Geometry: final body of the model. Coordinates: model frame, mm. Face numbers are marked on the shaded views. A direction names the side the tool comes from. Give positions to 0.01 mm unless a question says otherwise; leave off trailing zeros. Loops run counter-clockwise (first coordinate to the right, second up) from the corner with the lowest first, then second, coordinate; pieces in that order, holes last. Notation, with made-up numbers: (66.25, 24) - (79.25, 24) arc R24 cw to (79.25, 63) - close; hole circle Ø7 at (-9, 83). An arc over 180 degrees is marked (long way). Answer in a Markdown table with one row per item.
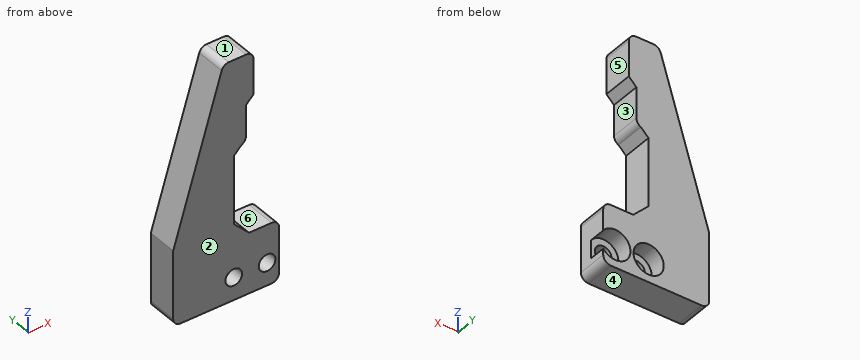
from build123d import *

# Parameters (mm, degrees)
BOSS_EXTRUDE1_DEPTH                                 = 10
CHAMFER1_SIZE                                       = 5
CHAMFER2_SIZE                                       = 2.5
FILLET1_R                                           = 2.5
CBORE_FOR_M5_HEX_SOCKET_HEAD_CAP_SCREW2_D           = 5.5
CBORE_FOR_M5_HEX_SOCKET_HEAD_CAP_SCREW2_DEPTH       = 10
CBORE_FOR_M5_HEX_SOCKET_HEAD_CAP_SCREW2_CBORE_D     = 10
CBORE_FOR_M5_HEX_SOCKET_HEAD_CAP_SCREW2_CBORE_DEPTH = 5.4
CBORE_FOR_M5_HEX_SOCKET_HEAD_CAP_SCREW2_TIP         = 1.652366702


# Some blends are built 0.0001 mm under size
with BuildPart() as part:
    # Sketch2 → Boss-Extrude1 (new body)
    with BuildSketch(Plane(origin=(0, 0, 0), x_dir=(1, 0, 0), z_dir=(0, 1, 0))):
        Polygon((0, 59.135462652), (-14.95, 59.135462652), (-14.95, 29.135462652), (-10.95, 29.135462652), (-10.95, 14.135462652), (-8.45, 14.135462652), (-8.45, 0), (-18.45, 0), (-35, 54.135462652), (-35, 79.135462652), (0, 79.135462652), align=None)
    extrude(amount=BOSS_EXTRUDE1_DEPTH)

    # Chamfer1
    chamfer1_edges = [part.edges().sort_by_distance(p)[0] for p in [
        (-14.95, 5, -59.135462652),
    ]]
    chamfer(chamfer1_edges, length=CHAMFER1_SIZE)

    # Chamfer2
    chamfer2_edges = [part.edges().sort_by_distance(p)[0] for p in [
        (-10.95, 5, -14.135462652),
        (-14.95, 5, -29.135462652),
    ]]
    chamfer(chamfer2_edges, length=CHAMFER2_SIZE - 0.0001)  # a hair under: the kernel refuses the full size

    # Fillet1
    # the kernel refuses this fillet: 2.5 mm, written as the material it takes off along each edge
    with BuildSketch(Plane(origin=(0, -6.25, -79.135462652), x_dir=(0, 0, 1), z_dir=(0, 1, 0)), Plane(origin=(-35, -6.25, -79.135462652), x_dir=(1, 0, 0), z_dir=(0, 1, 0)), Plane(origin=(0, -6.25, -59.135462652), x_dir=(-1, 0, 0), z_dir=(0, 1, 0))) as fillet1_piece_1:
        with BuildLine():
            CenterArc((FILLET1_R, -FILLET1_R), FILLET1_R, 90, 90)
            Line((0, -FILLET1_R), (-FILLET1_R * 0.02, -FILLET1_R))
            Line((-FILLET1_R * 0.02, -FILLET1_R), (-FILLET1_R * 0.02, FILLET1_R * 0.02))
            Line((-FILLET1_R * 0.02, FILLET1_R * 0.02), (FILLET1_R, FILLET1_R * 0.02))
            Line((FILLET1_R, FILLET1_R * 0.02), (FILLET1_R, 0))
        make_face()
    extrude(amount=22.5, mode=Mode.SUBTRACT)
    with BuildSketch(Plane(origin=(-8.45, -6.25, 0), x_dir=(0, 0, -1), z_dir=(0, 1, 0))) as fillet1_piece_2:
        with BuildLine():
            CenterArc((FILLET1_R, FILLET1_R), FILLET1_R, 180, 90)
            Line((0, FILLET1_R), (-FILLET1_R * 0.02, FILLET1_R))
            Line((-FILLET1_R * 0.02, FILLET1_R), (-FILLET1_R * 0.02, -FILLET1_R * 0.02))
            Line((-FILLET1_R * 0.02, -FILLET1_R * 0.02), (FILLET1_R, -FILLET1_R * 0.02))
            Line((FILLET1_R, -FILLET1_R * 0.02), (FILLET1_R, 0))
        make_face()
    extrude(amount=22.5, mode=Mode.SUBTRACT)
    with BuildSketch(Plane(origin=(-18.45, -4.62482795, 0), x_dir=(-0.29235761927834925, 0, -0.9563090622021188), z_dir=(0, 1, 0))) as fillet1_piece_3:
        with BuildLine():
            CenterArc((FILLET1_R * 0.739972471966, -FILLET1_R), FILLET1_R, 90, 73.00084391)
            Line((-FILLET1_R * 0.216336590236, -FILLET1_R * 0.707642380722), (-FILLET1_R * 0.23546277148, -FILLET1_R * 0.701795228336))
            Line((-FILLET1_R * 0.23546277148, -FILLET1_R * 0.701795228336), (-FILLET1_R * 0.0147994494393, FILLET1_R * 0.02))
            Line((-FILLET1_R * 0.0147994494393, FILLET1_R * 0.02), (FILLET1_R * 0.739972471966, FILLET1_R * 0.02))
            Line((FILLET1_R * 0.739972471966, FILLET1_R * 0.02), (FILLET1_R * 0.739972471966, 0))
        make_face()
    extrude(amount=19.2496559, mode=Mode.SUBTRACT)
    with BuildSketch(Plane(origin=(-10.95, -5.728328721, -29.135462652), x_dir=(-1, 0, 0), z_dir=(0, 1, 0))) as fillet1_piece_4:
        with BuildLine():
            CenterArc((2.5, 2.291331488), FILLET1_R, 180, 66.424322091)
            Line((0, 2.291331488), (-0.05, 2.291331488))
            Line((-0.05, 2.291331488), (-0.05, 0))
            Line((-0.05, 0), (0, -0.05))
            ThreePointArc((0, -0.05), (0.75005, -0.05), (1.480102, -0.04582663))
            Line((1.480102, -0.04582663), (1.5001, 0))
        make_face()
    extrude(amount=21.456657442, mode=Mode.SUBTRACT)

    # CBORE for M5 Hex Socket Head Cap Screw2
    with Locations(Plane(origin=(0, 10, 0), x_dir=(1, 0, 0), z_dir=(0, 1, 0))):
        with Locations((-15, 71.635462652), (-4, 71.635462652)):
            CounterBoreHole(CBORE_FOR_M5_HEX_SOCKET_HEAD_CAP_SCREW2_D / 2, CBORE_FOR_M5_HEX_SOCKET_HEAD_CAP_SCREW2_CBORE_D / 2, CBORE_FOR_M5_HEX_SOCKET_HEAD_CAP_SCREW2_CBORE_DEPTH, depth=CBORE_FOR_M5_HEX_SOCKET_HEAD_CAP_SCREW2_DEPTH)
            with Locations((0, 0, -(CBORE_FOR_M5_HEX_SOCKET_HEAD_CAP_SCREW2_DEPTH + CBORE_FOR_M5_HEX_SOCKET_HEAD_CAP_SCREW2_TIP / 2))):  # 118° drill point
                Cone(0, CBORE_FOR_M5_HEX_SOCKET_HEAD_CAP_SCREW2_D / 2, CBORE_FOR_M5_HEX_SOCKET_HEAD_CAP_SCREW2_TIP, mode=Mode.SUBTRACT)


solid = part.part
Q1. First-contact query: pin 1 (7 mm diameter, centred on x = -4, z = -72.5, fed in from +Y); pin 2 (3 mm diameter, centred on y = 3, z = -38.5, fed in from +X); pin 3 (6 mm diameter, centred on x = -6.5, y = 3.5, fed in from +Z); pin 4 (3.5 mm diameter, centred on x = -4, z = -71.64, fed in from +Y). Flat tips, straight axial feed; report the tip coordinate or a pass-through.
Check values:
| item | result |
|---|---|
| pin 1 | y = 4.6 |
| pin 2 | x = -14.95 |
| pin 3 | z = -0.46 |
| pin 4 | through |
Q2. Reachability of the marked faces 4, 5 and 6 from +Z, -Z, +X, -X, +Y, -Y: full face, straight path, thin tool, end or side. Return the list, or none.
Check values:
| item | result |
|---|---|
| face 4 | -Z, +X, -X, +Y, -Y |
| face 5 | +Z, +X, +Y, -Y |
| face 6 | +X, +Y, -Y |
Q3. Material intervals for line 1 along Z through (x, y) = (-15, 7.9); line 2 along Z through (x, y) = (-15, 2.6); line 3 along Z through (x, y) = (-11.5, 7.25), sorted ascending.
Check values:
| item | result |
|---|---|
| line 1 | -79.14 to -76.64, -66.64 to 0 |
| line 2 | -79.14 to -74.39, -68.89 to 0 |
| line 3 | -79.14 to -75.21, -68.06 to -57.59, -28.41 to 0 |
Q4. Cut plane A-A (x = -4). Output: boundary loops of the cut face in (y, z).
Check values:
| item | result |
|---|---|
| outline | (0, -79.14) - (10, -79.14) - (10, -76.64) - (4.6, -76.64) - (4.6, -74.39) - (0, -74.39) - close; (0, -68.89) - (4.6, -68.89) - (4.6, -66.64) - (10, -66.64) - (10, -59.14) - (0, -59.14) - close |
Q5. Cut plane C-C (z = -57). Output: boundary loops of the cut face in (x, y), and give its area (3 significant figures).
Check values:
| item | result |
|---|---|
| outline | (-35, 0) - (-12.09, 0) - (-12.09, 10) - (-35, 10) - close |
| area | 229 mm² |
Q6. Draft query along Z for the marked faces 1, 2 and 3. Return one class per face: pulls with the +Z half, pulls with the -Z half, needs draft (parallel to the pull), parting line crosses it, or undercut.
Check values:
| item | result |
|---|---|
| face 1 | pulls with the +Z half |
| face 2 | needs draft |
| face 3 | undercut |
Q7. Cut plane D-D (x = -30.5). Output: boundary loops of the cut face in (y, z), and give its area (3 significant figures).
Check values:
| item | result |
|---|---|
| outline | (0, -79.14) - (10, -79.14) - (10, -39.42) - (0, -39.42) - close |
| area | 397 mm² |
